Input: part model. Units: mm. Frame: model coordinates. Face numbers are marked on the shaded views. Coordinates: 2 decimals unless noted, no trailing zeros. Order: outer loops, then holes, each group sorted by start corner. A loop starts at its lowest first (then second) coordinate and runs counter-clockwise, first axis right, second up. Notation, with made-up numbers: (38, 57) - (48, 57) arc R15 cw to (48, 82) - close; hole circle Ø6 at (-8, 58.25). An arc over 180 degrees is marked (long way). Answer as CSV lines item,"result". Start each with the question number.
Item 1: Section B-B (z = 0). Output: boundary loops of the cut face in (x, y), and give its area (3 significant figures).
Item 2: Material intervals for line 1 along Z through (x, y) = (1.5, 10.5) (1 decimal); line 2 along Y through (x, z) = (-13, -1.5); line 3 along X through (y, z) = (81.5, 8), sorted ascending.
Item 3: Draft query along Z for the marked faces 1, 2 and 3. Return one class per face: +Z half, -Z half, draft (parallel to the pull), parting line (faces both ways), or undercut.
Item 4: Section C-C (y = 119.5). Output: boundary loops of the cut face in (x, z).
Item 5: First-contact query: pin 1 (12 mm diameter, centred on x = 16.5, y = 70.5, fed in from -Z); pin 2 (3 mm diameter, centred on y = 99, z = 11, fed in from +X); pin 3 (1.5 mm diameter, centred on y = 24.5, z = 9, fed in from -X). Flat tips, straight axial feed; report the tip coordinate or a pass-through.
Item 6: Section A-A (x = 0). Output: boundary loops of the cut face in (y, z).
Autodesk Inventor part; units mm, degrees
ref_plane "YZ Plane" through (0, 0, 0) normal (1, 0, 0) x (0, 1, 0)
ref_plane "XZ Plane" through (0, 0, 0) normal (0, 1, 0) x (-1, 0, 0)
ref_plane "XY Plane" through (0, 0, 0) normal (0, 0, 1) x (1, 0, 0)
sketch "Sketch1" plane through (0, 0, 0) normal (0, 1, 0) x (-1, 0, 0)
  circle A0 centre (0, 0) radius 50
  dimension "d0" = 100
extrude "Extrusion1" add sketch "Sketch1" along normal blind 140
shell "Shell1" thickness 5 removed faces 1 at (-9.39, 140, -8.8667)
fillet "Fillet1" radius 2 2 edges at (50, 0, 0) (45, 5, 0)
properties part number "Outer Layer"
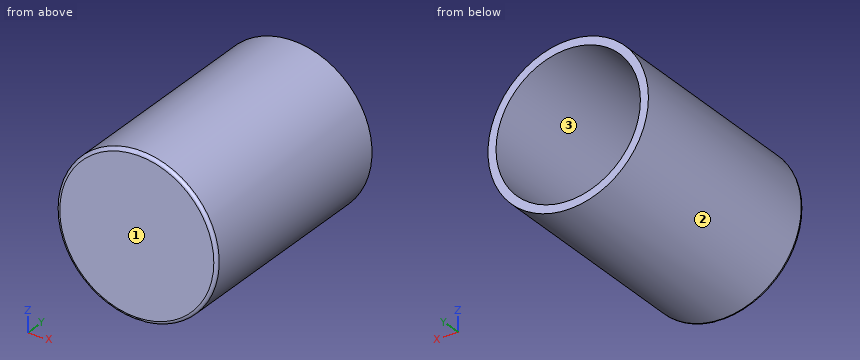
Determined:
1,outline,"(-50, 2) arc R2 ccw to (-48, 0) - (48, 0) arc R2 ccw to (50, 2) - (50, 140) - (45, 140) - (45, 7) arc R2 cw to (43, 5) - (-43, 5) arc R2 cw to (-45, 7) - (-45, 140) - (-50, 140) - close"
1,area,"1,850 mm^2"
2,line 1,"z = -50 to -45, 45 to 50"
2,line 2,"y = 0 to 5"
2,line 3,"x = -49.36 to -44.28, 44.28 to 49.36"
3,face 1,"draft"
3,face 2,"parting line"
3,face 3,"undercut"
4,outline,"circle Ø100 at (0, 0); hole circle Ø90 at (0, 0)"
5,pin 1,"stops at z = -48.89"
5,pin 2,"stops at x = 49.09"
5,pin 3,"stops at x = -49.31"
6,outline,"(0, -48) arc R2 ccw to (2, -50) - (140, -50) - (140, -45) - (7, -45) arc R2 cw to (5, -43) - (5, 43) arc R2 cw to (7, 45) - (140, 45) - (140, 50) - (2, 50) arc R2 ccw to (0, 48) - close"
